```python
from build123d import *

# Parameters (mm, degrees)
SKETCH_W        = 151
SKETCH_H        = 44
PAD_DEPTH       = 2
SKETCH001_W     = 161
SKETCH001_H     = 54
PAD001_DEPTH    = 2
SKETCH002_W     = 21
SKETCH002_H     = 27
PAD002_DEPTH    = 2
SKETCH003_W     = 15
SKETCH003_H     = 21
POCKET_DEPTH    = 3
SKETCH004_W     = 10.191287
SKETCH004_H     = 16.176647
POCKET001_DEPTH = 3.001
CHAMFER_SIZE    = 5
FILLET_R        = 5
FILLET001_R     = 3
CHAMFER001_SIZE = 1.9
SKETCH005_R     = 12
PAD003_DEPTH    = 2
SKETCH006_R     = 8
POCKET002_DEPTH = 2
CHAMFER002_SIZE = 1.9
SKETCH007_R     = 12
PAD004_DEPTH    = 2
POCKET003_DEPTH = 6.001
SKETCH009_W     = 80
SKETCH009_H     = 36
SKETCH009_W_2   = 71
SKETCH009_H_2   = 25
PAD005_DEPTH    = 2
FILLET002_R     = 5
SKETCH010_W     = 71
SKETCH010_H     = 25
POCKET004_DEPTH = 6.001
FILLET003_R     = 1.9
SKETCH011_W     = 85
SKETCH011_H     = 40
SKETCH011_W_2   = 81
SKETCH011_H_2   = 36
PAD006_DEPTH    = 2
SKETCH012_W     = 42
SKETCH012_H     = 5.5
POCKET005_DEPTH = 2
SKETCH013_W     = 5
SKETCH013_H     = 16
POCKET006_DEPTH = 3
SKETCH014_W     = 14.191287
SKETCH014_H     = 20.176647
SKETCH014_W_2   = 10.191287
SKETCH014_H_2   = 16.176647
PAD007_DEPTH    = 2


with BuildPart() as part:
    # Sketch → Pad (new body)
    with BuildSketch(Plane.XY):
        with Locations((75.5, 22)):
            Rectangle(SKETCH_W, SKETCH_H)
    extrude(amount=PAD_DEPTH)

    # Sketch001 (on Face6 of Pad) → Pad001 (join)
    with BuildSketch(Plane.XY.offset(2)):
        with Locations((75.5, 22)):
            Rectangle(SKETCH001_W, SKETCH001_H)
    extrude(amount=PAD001_DEPTH)

    # Sketch002 (on Face11 of Pad001) → Pad002 (join)
    with BuildSketch(Plane.XY.offset(4)):
        with Locations((15.5, 22)):
            Rectangle(SKETCH002_W, SKETCH002_H)
    extrude(amount=PAD002_DEPTH)

    # Sketch003 (on Face16 of Pad002) → Pocket (cut)
    with BuildSketch(Plane.XY.offset(6)):
        with Locations((15.5, 22)):
            Rectangle(SKETCH003_W, SKETCH003_H)
    extrude(amount=-POCKET_DEPTH, mode=Mode.SUBTRACT)

    # Sketch004 (on Face21 of Pocket) → Pocket001 (cut, through all)
    with BuildSketch(Plane.XY.offset(3)):
        with Locations((15.416752, 21.925829)):
            Rectangle(SKETCH004_W, SKETCH004_H)
    extrude(amount=-POCKET001_DEPTH, mode=Mode.SUBTRACT)

    # Chamfer
    chamfer_edges = [part.edges().sort_by_distance(p)[0] for p in [
        (151, 0, 1),
        (151, 44, 1),
        (0, 44, 1),
        (0, 0, 1),
    ]]
    chamfer(chamfer_edges, length=CHAMFER_SIZE)

    # Fillet
    fillet_edges = [part.edges().sort_by_distance(p)[0] for p in [
        (-5, -5, 3),
        (-5, 49, 3),
        (156, -5, 3),
        (156, 49, 3),
    ]]
    fillet(fillet_edges, radius=FILLET_R)

    # Fillet001
    fillet001_edges = [part.edges().sort_by_distance(p)[0] for p in [
        (26, 8.5, 5),
        (26, 35.5, 5),
        (5, 8.5, 5),
        (5, 35.5, 5),
    ]]
    fillet(fillet001_edges, radius=FILLET001_R)

    # Chamfer001
    chamfer001_edges = [part.edges().sort_by_distance(p)[0] for p in [
        (5, 22, 6),
    ]]
    chamfer(chamfer001_edges, length=CHAMFER001_SIZE)

    # Sketch005 (on Face4 of Chamfer001) → Pad003 (join)
    with BuildSketch(Plane.XY.offset(4)):
        with Locations((134, 22)):
            Circle(SKETCH005_R)
    extrude(amount=PAD003_DEPTH)

    # Sketch006 (on Face33 of Pad003) → Pocket002 (cut)
    with BuildSketch(Plane.XY.offset(6)):
        with Locations((134, 22)):
            Circle(SKETCH006_R)
    extrude(amount=-POCKET002_DEPTH, mode=Mode.SUBTRACT)

    # Chamfer002
    chamfer002_edges = [part.edges().sort_by_distance(p)[0] for p in [
        (122, 22, 6),
    ]]
    chamfer(chamfer002_edges, length=CHAMFER002_SIZE)

    # Sketch007 (on Face41 of Chamfer002) → Pad004 (join)
    with BuildSketch(Plane(origin=(0, 0, 0), x_dir=(1, 0, 0), z_dir=(0, 0, -1))):
        with Locations((134, -22)):
            Circle(SKETCH007_R)
    extrude(amount=PAD004_DEPTH)

    # Sketch008 (on Face31 of Pad004) → Pocket003 (cut, through all)
    with BuildSketch(Plane.XY.offset(4)):
        with BuildLine():
            ThreePointArc((131.938447, 26), (129.5, 22), (131.938447, 18))
            Line((136.061553, 18), (131.938447, 18))
            ThreePointArc((136.061553, 18), (138.5, 22), (136.061553, 26))
            Line((131.938447, 26), (136.061553, 26))
        make_face()
    extrude(amount=-POCKET003_DEPTH, mode=Mode.SUBTRACT)

    # Sketch009 (on Face3 of Pocket003) → Pad005 (join)
    with BuildSketch(Plane.XY.offset(4)):
        with Locations((75.5, 22)):
            Rectangle(SKETCH009_W, SKETCH009_H)
        with Locations((75.5, 22)):
            Rectangle(SKETCH009_W_2, SKETCH009_H_2, mode=Mode.SUBTRACT)
    extrude(amount=PAD005_DEPTH)

    # Fillet002
    fillet002_edges = [part.edges().sort_by_distance(p)[0] for p in [
        (115.5, 4, 5),
        (115.5, 40, 5),
        (35.5, 4, 5),
        (35.5, 40, 5),
    ]]
    fillet(fillet002_edges, radius=FILLET002_R)

    # Sketch010 (on Face52 of Fillet002) → Pocket004 (cut, through all)
    with BuildSketch(Plane.XY.offset(4)):
        with Locations((75.5, 22)):
            Rectangle(SKETCH010_W, SKETCH010_H)
    extrude(amount=-POCKET004_DEPTH, mode=Mode.SUBTRACT)

    # Fillet003
    fillet003_edges = [part.edges().sort_by_distance(p)[0] for p in [
        (75.5, 40, 6),
    ]]
    fillet(fillet003_edges, radius=FILLET003_R)

    # Sketch011 (on Face64 of Fillet003) → Pad006 (join)
    with BuildSketch(Plane(origin=(0, 0, 0), x_dir=(1, 0, 0), z_dir=(0, 0, -1))):
        with Locations((75.5, -22)):
            Rectangle(SKETCH011_W, SKETCH011_H)
        with Locations((75.5, -22)):
            Rectangle(SKETCH011_W_2, SKETCH011_H_2, mode=Mode.SUBTRACT)
    extrude(amount=PAD006_DEPTH)

    # Sketch012 (on Face64 of Pad006) → Pocket005 (cut)
    with BuildSketch(Plane(origin=(0, 0, 0), x_dir=(1, 0, 0), z_dir=(0, 0, -1))):
        with Locations((90, -6.75)):
            Rectangle(SKETCH012_W, SKETCH012_H)
        with Locations((61, -37.25)):
            Rectangle(SKETCH012_W, SKETCH012_H)
    extrude(amount=-POCKET005_DEPTH, mode=Mode.SUBTRACT)

    # Sketch013 (on Face68 of Pocket005) → Pocket006 (cut)
    with BuildSketch(Plane(origin=(0, 0, 0), x_dir=(1, 0, 0), z_dir=(0, 0, -1))):
        with Locations((37.5, -22)):
            Rectangle(SKETCH013_W, SKETCH013_H)
        with Locations((113.5, -22)):
            Rectangle(SKETCH013_W, SKETCH013_H)
    extrude(amount=-POCKET006_DEPTH, mode=Mode.SUBTRACT)

    # Sketch014 (on Face80 of Pocket006) → Pad007 (join)
    with BuildSketch(Plane(origin=(0, 0, 0), x_dir=(1, 0, 0), z_dir=(0, 0, -1))):
        with Locations((15.416752, -21.925829)):
            Rectangle(SKETCH014_W, SKETCH014_H)
        with Locations((15.416752, -21.925829)):
            Rectangle(SKETCH014_W_2, SKETCH014_H_2, mode=Mode.SUBTRACT)
    extrude(amount=PAD007_DEPTH)


solid = part.part
```
Geometry: final body of the model. Coordinates: model frame, mm. A direction names the side the tool comes from. Coordinates: 2 decimals unless noted, no trailing zeros. Loops run counter-clockwise (first coordinate to the right, second up) from the corner with the lowest first, then second, coordinate; pieces in that order, holes last. Notation, with made-up numbers: (23, 21.5) -> (51, 21.5) arc R15 ccw to (51, 29.5) -> close; hole circle Ø8 at (1.25, 35.25). An arc over 180 degrees is marked (long way). Use a Markdown table: item, result. Add a question column.
(1) Access query for faces 4 (the conical face through (6.544, 33.924, 5.063)), 5 (the flat face through (37, 22, 3)), 6 (the flat face through (137.4, 18.6, 4)), 7 (the flat face through (149, 3, 1)). Directions: +Z, -Z, +X, -X, +Y, -Y. A direction counts if a zero-diameter tool reaches every point of the face in a straight line with its end or side. Return the directions, or none.
(2) Mould query, pull axis Y, two halves, no side actions, for faces 1 (the conical face through (24.424, 33.956, 5.063)), 2 (the flat face through (61, 37, 2)), 3 (the flat face through (78, 9, 6)). Classes: pulls with the +Y half, pulls with the -Y half, needs draft (parallel to the pull), parting line crosses it, or undercut.
(3) Line query: line 1 along X through (y, z) = (14.5, 2.75); line 2 along Y through (x, z) = (11, -1.5); line 3 along Y through (x, z) = (46, 3.25). Output: solid intervals per line, ascending.
(4) Pin query (flat end, axial travel): pin 1 Ø4 at (x, y) = (30, 21) entering from -Z; pin 2 Ø0.9 at (x, z) = (113, 1.5) entering from -Y; pin 3 Ø0.6 at (x, z) = (15.5, -1) entering from -Y. Return the tip coordinate at first contact, or that it passes through.
(5) Section query A-A, the plane x = 134. Return loops of the section in (y, z).
(6) Section query C-C, the plane x = 77.5. Return loops of the section in (y, z), plus the area to 3 significant figures.
(7) Section query B-B, the plane y = 22. State how many separate pieces and enclosed holes the cut face has, plus the area to 3 significant figures.
Answer:
| question | item | result |
|---|---|---|
| 1 | face 4 | +Z, -X, +Y |
| 1 | face 5 | -Z |
| 1 | face 6 | +Z |
| 1 | face 7 | -Z, +X, -Y |
| 2 | face 1 | pulls with the +Y half |
| 2 | face 2 | undercut |
| 2 | face 3 | needs draft |
| 3 | line 1 | x = -5 to 10.32, 20.51 to 35, 116 to 156 |
| 3 | line 2 | y = 11.84 to 13.84, 30.01 to 32.01 |
| 3 | line 3 | y = -5 to 9.5, 34.5 to 49 |
| 4 | pin 1 | stops at z = 0 |
| 4 | pin 2 | stops at y = 0 |
| 4 | pin 3 | stops at y = 11.84 |
| 5 | outline | (-5, 2) -> (0, 2) -> (0, 0) -> (10, 0) -> (10, -2) -> (18, -2) -> (18, 4) -> (14, 4) -> (14, 6) -> (11.9, 6) -> (10, 4.1) -> (10, 4) -> (-5, 4) -> close; (26, -2) -> (34, -2) -> (34, 0) -> (44, 0) -> (44, 2) -> (49, 2) -> (49, 4) -> (34, 4) -> (34, 4.1) -> (32.1, 6) -> (30, 6) -> (30, 4) -> (26, 4) -> close |
| 6 | outline | (-5, 2) -> (0, 2) -> (0, 0) -> (2, 0) -> (2, -2) -> (4, -2) -> (4, 2) -> (9.5, 2) -> (9.5, 6) -> (5.9, 6) arc R1.9 ccw to (4, 4.1) -> (4, 4) -> (-5, 4) -> close; (34.5, 2) -> (40, 2) -> (40, -2) -> (42, -2) -> (42, 0) -> (44, 0) -> (44, 2) -> (49, 2) -> (49, 4) -> (40, 4) -> (40, 4.1) arc R1.9 ccw to (38.1, 6) -> (34.5, 6) -> close |
| 6 | area | 102 mm^2 |
| 7 | separate pieces | 4 |
| 7 | enclosed holes | 0 |
| 7 | area | 312 mm^2 |
